from build123d import *

# Parameters (mm, degrees)
SKETCH4_R           = 28
SKETCH4_R_2         = 25
EXTRUDE_THIN2_DEPTH = 5


# Read off the part's stored shape, not the designer's step: Shell1
with BuildPart() as part:
    # Sketch1 → Revolve1 (revolve)
    with BuildSketch(Plane.XY, mode=Mode.PRIVATE) as revolve1_sk:
        with BuildLine():
            Line((0, 0), (0, 100))
            Line((0, 100), (30, 100))
            Line((30, 100), (30, 54.403065089))
            ThreePointArc((30, 54.403065089), (29.682011865, 50.046670749), (28.734788557, 45.782628522))
            Line((28.734788557, 45.782628522), (15, 0))
            Line((15, 0), (0, 0))
        make_face()
    revolve(revolve1_sk.sketch.rotate(Axis((0, 0, 0), (0, 1, 0)), 90), axis=Axis((0, 0, 0), (0, 1, 0)))

    # Sketch4 → Extrude-Thin2 (add)
    with BuildSketch(Plane(origin=(0, 100, 0), x_dir=(1, 0, 0), z_dir=(0, 1, 0))):
        Circle(SKETCH4_R)
        Circle(SKETCH4_R_2, mode=Mode.SUBTRACT)
    extrude(amount=EXTRUDE_THIN2_DEPTH)

    # Shell1 outline → Shell1 (revolve, cut)
    with BuildSketch(Plane.XY):
        with BuildLine():
            Line((25, 97), (25, 100))
            Line((25, 100), (0, 100))
            Line((0, 100), (0, 3))
            Line((0, 3), (12.767908047, 3))
            Line((12.767908047, 3), (25.861309693, 46.644672153))
            ThreePointArc((25.861309693, 46.644672153), (26.713810678, 50.482310183), (27, 54.403065116))
            Line((27, 54.403065116), (27, 97))
            Line((27, 97), (25, 97))
        make_face()
    revolve(axis=Axis((0, 0, 0), (0, 1, 0)), mode=Mode.SUBTRACT)


solid = part.part
Could you check a few things on this model? Use its own coordinates, in mm. A direction names the side the tool comes from. Coordinates: 2 decimals unless noted, no trailing zeros. Write each loop counter-clockwise with the first axis right and the second up, starting at its lowest first coordinate (ties: lowest second). Pieces come first, ordered by that corner, then holes. Notation, with made-up numbers: (87.5, -6.75) - (140.5, -6.75) arc R24 cw to (140.5, 27.25) - close; hole circle Ø8 at (-7, 18.25). An arc over 180 degrees is marked (long way). Put each result on its own line as item: value. Start each with the question number.
Q1. Which directions (+Z, -Z, +X, -X, +Y, -Y) give clear straight access to the entire face, cutting with the end or side of a thin tool? Please do faces 1 (the cylindrical face through (-5.85, 76, 26.36)), 2 (the cylindrical face through (-25.296, 76.882, -16.128)), 3 (the cylindrical face through (23.846, 100.944, -7.509)).
Q2. I want a section at C-C on y = 43.5. Write out the boundary of the cut face in (x, z).
Q3. I want a section at B-B on z = 0. Write out the boundary of the cut face in (x, y).
Q4. Please list where these lines run through material, in increasing order: L1, parallel to X at y = 81, z = 0; L2, parallel to Z at x = 0, y = 101.
Q5. I'm going to push flat-ended pins straight in: P1, Ø3, axis at y = 26, z = -15, coming from the -X side; P2, Ø3, axis at x = -2, y = 89.5, coming from the -Z side; P3, Ø10, axis at y = 44, z = -4, coming from the +X side. Where does each tip first touch, or does it pass through?
Q6. I want a section at A-A on x = 0. Write out the boundary of the cut face in (y, z), plus the area to 3 significant figures.
Q7. Thinking about a two-plate mould opening in X: for faces 4 (the flat face through (0, 3, 0)), 5 (the flat face through (0, 0, 0)), 6 (the cylindrical face through (25.865, 102.465, 10.724)), which applies, pulls with the +X half, pulls with the -X half, needs draft (parallel to the pull), parting line crosses it, or undercut?
Q8. I want a section at D-D on y = 89.5. Write out the boundary of the cut face in (x, z), plus the area to 3 significant figures.
Checks:
1. face 1: none
1. face 2: +Y, -Y
1. face 3: +Y
2. outline: circle Ø56.1 at (0, 0); hole circle Ø49.84 at (0, 0)
3. outline: (-30, 54.4) arc R30 ccw to (-28.73, 45.78) - (-15, 0) - (15, 0) - (28.73, 45.78) arc R30 ccw to (30, 54.4) - (30, 100) - (28, 100) - (28, 105) - (25, 105) - (25, 97) - (27, 97) - (27, 54.4) arc R27 cw to (25.86, 46.64) - (12.77, 3) - (-12.77, 3) - (-25.86, 46.64) arc R27 cw to (-27, 54.4) - (-27, 97) - (-25, 97) - (-25, 105) - (-28, 105) - (-28, 100) - (-30, 100) - close
4. L1: -30 to -27, 27 to 30
4. L2: -28 to -25, 25 to 28
5. P1: x = -18.51
5. P2: z = -30
5. P3: x = 29.36
6. outline: (0, -15) - (45.78, -28.73) arc R30 ccw to (54.4, -30) - (100, -30) - (100, -28) - (105, -28) - (105, -25) - (97, -25) - (97, -27) - (54.4, -27) arc R27 cw to (46.64, -25.86) - (3, -12.77) - (3, 12.77) - (46.64, 25.86) arc R27 cw to (54.4, 27) - (97, 27) - (97, 25) - (105, 25) - (105, 28) - (100, 28) - (100, 30) - (54.4, 30) arc R30 ccw to (45.78, 28.73) - (0, 15) - close
6. area: 729 mm²
7. face 4: undercut
7. face 5: needs draft
7. face 6: parting line crosses it
8. outline: circle Ø60 at (0, 0); hole circle Ø54 at (0, 0)
8. area: 537 mm²
